```python
from build123d import *

# Parameters (mm, degrees)
SKETCH1_W               = 42.3
SKETCH1_H               = 42.3
BOSS_EXTRUDE1_DEPTH     = 20.5
SKETCH2_R               = 11
BOSS_EXTRUDE2_DEPTH     = 2
SKETCH3_R               = 2.5
BOSS_EXTRUDE3_DEPTH     = 16
CUT_EXTRUDE1_DEPTH      = 19
CUT_EXTRUDE1_DEPTH_BACK = 21.5
SKETCH5_W               = 33.814718626
SKETCH5_H               = 3.5
CUT_EXTRUDE2_DEPTH      = 0.01
CUT_EXTRUDE3_START      = -12
CUT_EXTRUDE3_DEPTH      = 3.5
CIRPATTERN1_COUNT       = 4
SKETCH7_R               = 1.5
CUT_EXTRUDE4_DEPTH      = 4.5
SKETCH8_W               = 16
SKETCH8_H               = 11
BOSS_EXTRUDE4_DEPTH     = 6
SKETCH9_W               = 16
SKETCH9_H               = 5
CUT_EXTRUDE5_DEPTH      = 2.5
FILLET1_R               = 1.5
SKETCH10_W              = 13
SKETCH10_H              = 4.5
CUT_EXTRUDE6_DEPTH      = 5
CUT_EXTRUDE7_DEPTH      = 30.15
BOSS_EXTRUDE5_DEPTH     = 4


with BuildPart() as part:
    # Sketch1 → Boss-Extrude1 (new body)
    with BuildSketch(Plane(origin=(0, 0, 0), x_dir=(1, 0, 0), z_dir=(0, 1, 0))):
        Rectangle(SKETCH1_W, SKETCH1_H)
    extrude(amount=BOSS_EXTRUDE1_DEPTH)

    # Sketch2 → Boss-Extrude2 (add)
    with BuildSketch(Plane(origin=(0, 20.5, 0), x_dir=(1, 0, 0), z_dir=(0, 1, 0))):
        Circle(SKETCH2_R)
    extrude(amount=BOSS_EXTRUDE2_DEPTH)

    # Sketch3 → Boss-Extrude3 (add)
    with BuildSketch(Plane(origin=(0, 22.5, 0), x_dir=(1, 0, 0), z_dir=(0, 1, 0))):
        Circle(SKETCH3_R)
    extrude(amount=BOSS_EXTRUDE3_DEPTH)

    # Sketch4 → Cut-Extrude1 (cut, two sides)
    with BuildSketch(Plane(origin=(0, 20.5, 0), x_dir=(1, 0, 0), z_dir=(0, 1, 0))) as cut_extrude1_sk:
        Polygon((-21.15, 16.907359313), (-16.907359313, 21.15), (-21.15, 21.15), align=None)
        Polygon((21.15, 21.15), (21.15, 16.907359313), (16.907359313, 21.15), align=None)
        Polygon((21.15, -16.907359313), (16.907359313, -21.15), (21.15, -21.15), align=None)
        Polygon((-21.15, -21.15), (-21.15, -16.907359313), (-16.907359313, -21.15), align=None)
    extrude(amount=CUT_EXTRUDE1_DEPTH, mode=Mode.SUBTRACT)
    extrude(cut_extrude1_sk.sketch, amount=-CUT_EXTRUDE1_DEPTH_BACK, mode=Mode.SUBTRACT)

    # Sketch5 → Cut-Extrude2 (cut)
    with BuildSketch(Plane(origin=(21.15, 0, 0), x_dir=(0, 0, -1), z_dir=(1, 0, 0))):
        with Locations((0, 10.25)):
            Rectangle(SKETCH5_W, SKETCH5_H)
    cut_extrude2 = extrude(amount=-CUT_EXTRUDE2_DEPTH, mode=Mode.SUBTRACT)

    # Sketch6 → Cut-Extrude3 (cut)
    with BuildSketch(Plane(origin=(0, 20.5, 0), x_dir=(1, 0, 0), z_dir=(0, 1, 0)).offset(CUT_EXTRUDE3_START)):
        Polygon((21.15, 14.078932188), (14.078932188, 21.15), (21.15, 21.15), align=None)
    cut_extrude3 = extrude(amount=CUT_EXTRUDE3_DEPTH, mode=Mode.SUBTRACT)

    # CirPattern1: Cut-Extrude2, Cut-Extrude3 ×4 about axis
    cirpattern1_axis = Axis((0, 0, 0), (0, 1, 0))
    for i in range(1, CIRPATTERN1_COUNT):
        add(cut_extrude2.rotate(cirpattern1_axis, i * 360 / CIRPATTERN1_COUNT), mode=Mode.SUBTRACT)
        add(cut_extrude3.rotate(cirpattern1_axis, i * 360 / CIRPATTERN1_COUNT), mode=Mode.SUBTRACT)

    # Sketch7 → Cut-Extrude4 (cut)
    with BuildSketch(Plane(origin=(0, 20.5, 0), x_dir=(1, 0, 0), z_dir=(0, 1, 0))):
        with Locations((15.5, 15.5)):
            Circle(SKETCH7_R)
        with Locations((15.5, -15.5)):
            Circle(SKETCH7_R)
        with Locations((-15.5, -15.5)):
            Circle(SKETCH7_R)
        with Locations((-15.5, 15.5)):
            Circle(SKETCH7_R)
    extrude(amount=-CUT_EXTRUDE4_DEPTH, mode=Mode.SUBTRACT)

    # Sketch8 → Boss-Extrude4 (add)
    with BuildSketch(Plane.XY.offset(21.15)):
        with Locations((0, 5.5)):
            Rectangle(SKETCH8_W, SKETCH8_H)
    extrude(amount=BOSS_EXTRUDE4_DEPTH)

    # Sketch9 → Cut-Extrude5 (cut)
    with BuildSketch(Plane.XY.offset(27.15)):
        with Locations((0, 2.5)):
            Rectangle(SKETCH9_W, SKETCH9_H)
    extrude(amount=-CUT_EXTRUDE5_DEPTH, mode=Mode.SUBTRACT)

    # Fillet1
    fillet1_edges = [part.edges().sort_by_distance(p)[0] for p in [
        (0, 0, 24.65),
    ]]
    fillet(fillet1_edges, radius=FILLET1_R)

    # Sketch10 → Cut-Extrude6 (cut)
    with BuildSketch(Plane(origin=(0, 11, 0), x_dir=(1, 0, 0), z_dir=(0, 1, 0))):
        with Locations((0, -24.9)):
            Rectangle(SKETCH10_W, SKETCH10_H)
    extrude(amount=-CUT_EXTRUDE6_DEPTH, mode=Mode.SUBTRACT)

    # Sketch11 → Cut-Extrude7 (cut, through all)
    with BuildSketch(Plane(origin=(8, 0, 0), x_dir=(0, 0, -1), z_dir=(1, 0, 0))):
        with BuildLine():
            Line((-27.15, 9.5), (-25.15, 9.5))
            ThreePointArc((-25.15, 9.5), (-24.65, 9), (-25.15, 8.5))
            Line((-25.15, 8.5), (-27.15, 8.5))
            Line((-27.15, 8.5), (-27.15, 9.5))
        make_face()
    extrude(amount=-CUT_EXTRUDE7_DEPTH, mode=Mode.SUBTRACT)

    # Sketch12 → Boss-Extrude5 (add)
    with BuildSketch(Plane(origin=(0, 6, 0), x_dir=(1, 0, 0), z_dir=(0, 1, 0))):
        with BuildLine():
            Line((-2.667, -22.65), (-2.167, -22.65))
            Line((-2.167, -22.65), (-2.167, -26.4))
            ThreePointArc((-2.167, -26.4), (-2.417, -26.65), (-2.667, -26.4))
            Line((-2.667, -26.4), (-2.667, -22.65))
        make_face()
        with BuildLine():
            Line((5.334, -22.65), (5.334, -26.4))
            ThreePointArc((5.334, -26.4), (5.084, -26.65), (4.834, -26.4))
            Line((4.834, -26.4), (4.834, -22.65))
            Line((4.834, -22.65), (5.334, -22.65))
        make_face()
        with BuildLine():
            Line((-4.834, -22.65), (-5.334, -22.65))
            Line((-5.334, -22.65), (-5.334, -26.4))
            ThreePointArc((-5.334, -26.4), (-5.084, -26.65), (-4.834, -26.4))
            Line((-4.834, -26.4), (-4.834, -22.65))
        make_face()
        with BuildLine():
            Line((2.167, -22.65), (2.167, -26.4))
            ThreePointArc((2.167, -26.4), (2.417, -26.65), (2.667, -26.4))
            Line((2.667, -26.4), (2.667, -22.65))
            Line((2.667, -22.65), (2.167, -22.65))
        make_face()
    extrude(amount=BOSS_EXTRUDE5_DEPTH)


solid = part.part
```
Input: part model. Units: mm. Frame: model coordinates. A direction names the side the tool comes from. Coordinates: 2 decimals unless noted, no trailing zeros. Loops run counter-clockwise (first coordinate to the right, second up) from the corner with the lowest first, then second, coordinate; pieces in that order, holes last. Notation, with made-up numbers: (80, 25.5) - (110, 25.5) arc R26 ccw to (110, 58.5) - close; hole circle Ø1 at (71.25, 57.25). An arc over 180 degrees is marked (long way). Answer in a Markdown table with one row per item.
(1) Material intervals for L1, parallel to X at y = 18.7, z = -15.5; L2, parallel to Z at x = -15, y = 17, sorted ascending. Write a range as from..to.
Model answer:
| item | result |
|---|---|
| L1 | x = -21.15..-17, -14..14, 17..21.15 |
| L2 | z = -21.15..-16.91, -14.09..14.09, 16.91..21.15 |
(2) Pin query (flat end, axial travel): P1, Ø4, axis at y = 8.5, z = 25, coming from the -X side; P2, Ø1.9, axis at y = 8, z = 23.5, coming from the +X side; P3, Ø1.5, axis at x = -5, z = 12.5, coming from the +Y side. Return the tip coordinate at first contact, or that it passes through.
Model answer:
| item | result |
|---|---|
| P1 | stops at x = -8 |
| P2 | stops at x = 8 |
| P3 | stops at y = 20.5 |
(3) Set-up query: faces 4 (the face through (-17.66, 10.23, 17.57)), 5 (the face through (12, 4, 21.15)), 6 (the face through (-6.5, 9, 24)). Return all of +Z, -Z, +X, -X, +Y, -Y with unobstructed straight access to the full face (end or side cutting, diameter ignored); none if empty.
Model answer:
| item | result |
|---|---|
| face 4 | +Z, -X |
| face 5 | +Z, +X, +Y, -Y |
| face 6 | +Z, +Y |
(4) Mould query, pull axis X, two halves, no side actions, for faces 1 (the face through (-17, 18.28, 15.43)), 2 (the face through (19.06, 4.31, 19)), 3 (the face through (-19.06, 4.31, -19)). Classes: pulls with the +X half, pulls with the -X half, needs draft (parallel to the pull), parting line crosses it, or undercut.
Model answer:
| item | result |
|---|---|
| face 1 | undercut |
| face 2 | pulls with the +X half |
| face 3 | pulls with the -X half |
(5) Cut plane C-C on y = 21.5. Output: boundary loops of the cut face in (x, z).
Model answer:
| item | result |
|---|---|
| outline | circle Ø22 at (0, 0) |
